Can you work these out from the drawing? Everything is in mm from the part's minimum corner. A direction names the side the tool comes from. Coordinates: 2 decimals unless noted, no trailing zeros. Write each loop counter-clockwise with the first axis right and the second up, starting at its lowest first coordinate (ties: lowest second). Pieces come first, ordered by that corner, then holes. Notation, with made-up numbers: (10.5, 5.5) -> (55.5, 5.5) arc R29 ccw to (55.5, 40.5) -> close; hole circle Ø9 at (-3, 78.25). An arc over 180 degrees is marked (long way). Use a Markdown table: item, result. Add a question column.
Item 1: If I drill on line 1 along Z through (x, y) = (2.5, 4.75); line 2 along Y through (x, z) = (7.5, 3.4); line 3 along X through (y, z) = (6.75, 3.5), over which ranges is the centre line in solid material (lowest first)? Write a range as from..to.
Item 2: On a 3-axis mill with a long thin cutter (end or side, diameter ignored), from which of +Z, -Z, +X, -X, +Y, -Y can I reach the whole of each face in a straight line? I mean the marked faces 1 and 2. Say none if no direction works.
Item 3: If we mould it in two halves opening along Y, with no side actions, what happens to the marked faces 3, 4 and 5? For each: pulls with the +Y half, pulls with the -Y half, needs draft (parallel to the pull), parting line crosses it, or undercut.
Item 4: Will these pins go through, and if not, where does the flat tip stop? pin 1 Ø2 at (x, z) = (5.5, 3) entering from -Y; pin 2 Ø1.3 at (x, y) = (7.5, 7.5) entering from -Z; pin 3 Ø1.8 at (x, y) = (8, 7) entering from -Z; pin 4 Ø1.5 at (y, z) = (6, 3) entering from +X.
Item 5: Imagine slicing it at C-C, the plane z = 2.5. Write out the boundary of the cut face in (x, y), and give its area (3 significant figures).
Item 6: Imagine slicing it at D-D, the plane z = 4.5. Write out the boundary of the cut face in (x, y).
Item 7: Imagine slicing it at A-A, the plane y = 7.5. Write out the boundary of the cut face in (x, z).
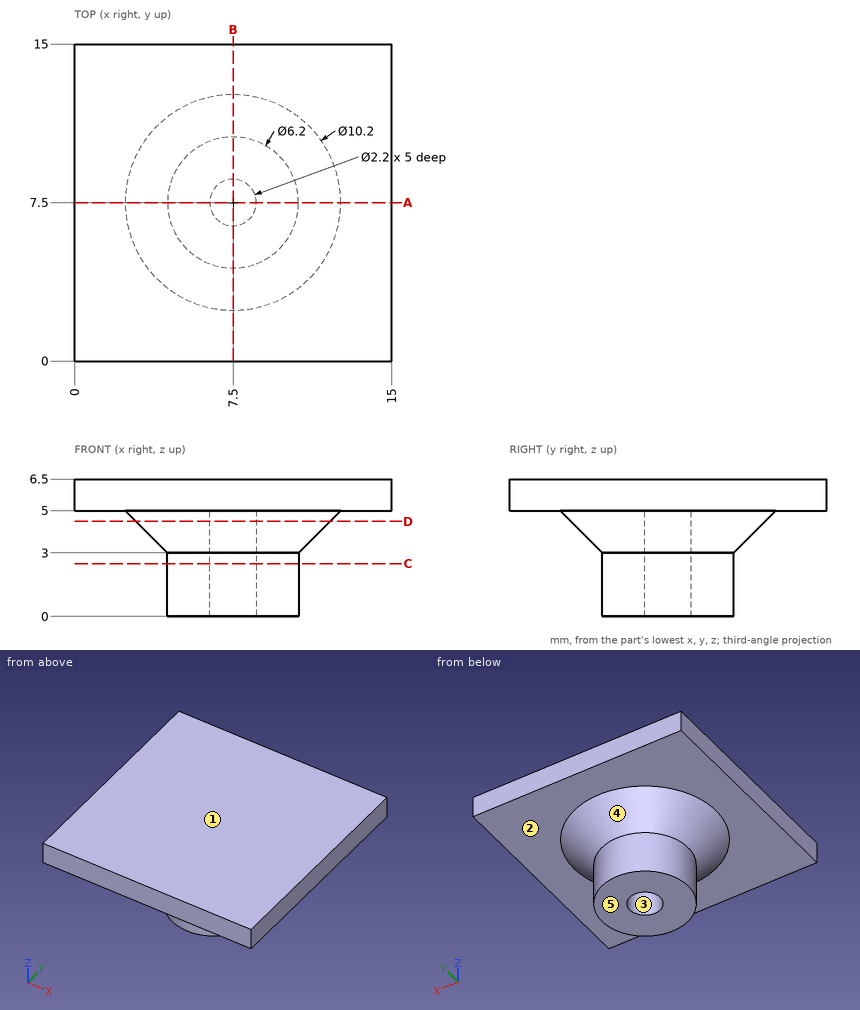
Ans:
| question | item | result |
|---|---|---|
| 1 | line 1 | z = 5..6.5 |
| 1 | line 2 | y = 4..6.4, 8.6..11 |
| 1 | line 3 | x = 3.98..6.7, 8.3..11.02 |
| 2 | face 1 | +Z, +X, -X, +Y, -Y |
| 2 | face 2 | -Z |
| 3 | face 3 | undercut |
| 3 | face 4 | parting line crosses it |
| 3 | face 5 | needs draft |
| 4 | pin 1 | stops at y = 3.82 |
| 4 | pin 2 | stops at z = 5 |
| 4 | pin 3 | stops at z = 0 |
| 4 | pin 4 | stops at x = 11.1 |
| 5 | outline | circle Ø6.2 at (7.5, 7.5); hole circle Ø2.2 at (7.5, 7.5) |
| 5 | area | 26.4 mm^2 |
| 6 | outline | circle Ø9.2 at (7.5, 7.5); hole circle Ø2.2 at (7.5, 7.5) |
| 7 | outline | (0, 5) -> (2.4, 5) -> (4.4, 3) -> (4.4, 0) -> (6.4, 0) -> (6.4, 5) -> (8.6, 5) -> (8.6, 0) -> (10.6, 0) -> (10.6, 3) -> (12.6, 5) -> (15, 5) -> (15, 6.5) -> (0, 6.5) -> close |
